Answer from the drawing. Dimensions are ordinates in mm from the lowest x, y and z of the part. Round coordinates to 2 decimals unless told otherwise and drop trailing zeros. Loops run counter-clockwise (first coordinate to the right, second up) from the corner with the lowest first, then second, coordinate; pieces in that order, holes last.
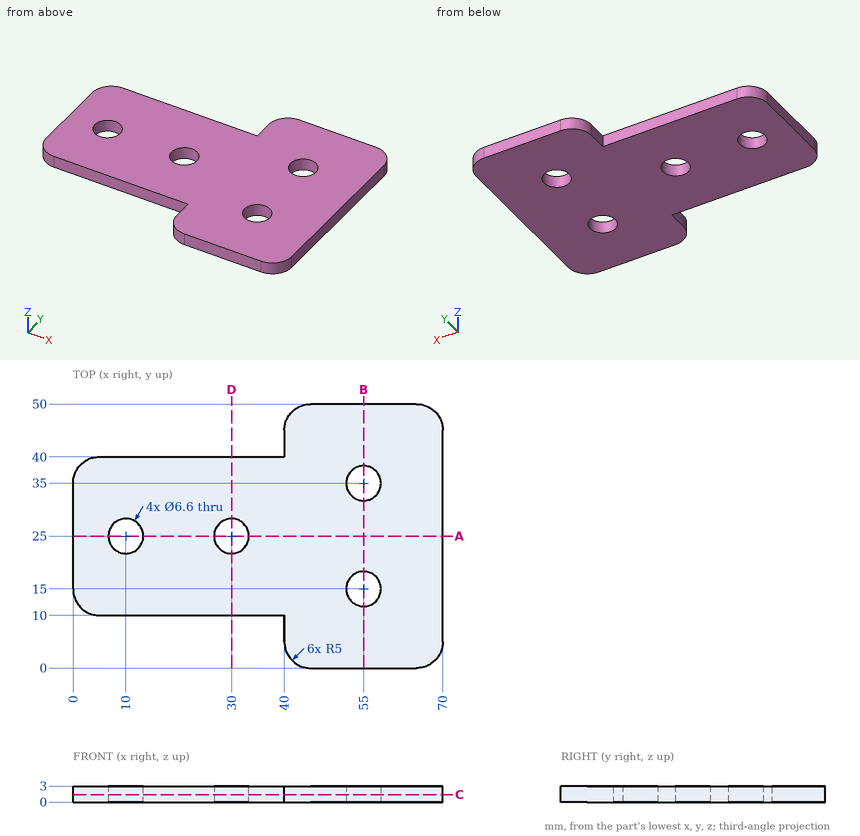
1. Find section D-D (x = 30). Write down the section's boundary in (y, z), then the cut area to 3 significant figures.
Answer key:
outline: (10, 0) - (21.7, 0) - (21.7, 3) - (10, 3) - close; (28.3, 0) - (40, 0) - (40, 3) - (28.3, 3) - close
area: 70.2 mm2
2. Find section A-A (y = 25). Write down the section's boundary in (x, z).
Answer key:
outline: (0, 0) - (6.7, 0) - (6.7, 3) - (0, 3) - close; (13.3, 0) - (26.7, 0) - (26.7, 3) - (13.3, 3) - close; (33.3, 0) - (70, 0) - (70, 3) - (33.3, 3) - close
3. Given pin 1 (10.5 mm diameter, centred on x = 55, y = 35, fed in from +Z); pin 2 (5.5 mm diameter, centred on x = 55, y = 15, fed in from -Z); pin 3 (1.5 mm diameter, centred on y = 7, z = 1, fed in from -X); pin 4 (1.5 mm diameter, centred on x = 17, z = 2.5, fed in from +Y), each flat-ended and moving along its own axis, determine where each tip first touches the part or whether it passes through.
Answer key:
pin 1: stops at z = 3
pin 2: passes through
pin 3: stops at x = 40
pin 4: stops at y = 40
4. Consider probe 1 along Y at (x, z) = (55, 1.1); probe 2 along Y at (x, z) = (10, 1.1); probe 3 along X at (y, z) = (28, 0.4). Determine where each line is inside the solid, lowest interval first.
Answer key:
probe 1: y = 0 to 11.7, 18.3 to 31.7, 38.3 to 50
probe 2: y = 10 to 21.7, 28.3 to 40
probe 3: x = 0 to 8.63, 11.37 to 28.63, 31.37 to 70
5. Find section B-B (x = 55). Write down the section's boundary in (y, z), then the cut area to 3 significant figures.
Answer key:
outline: (0, 0) - (11.7, 0) - (11.7, 3) - (0, 3) - close; (18.3, 0) - (31.7, 0) - (31.7, 3) - (18.3, 3) - close; (38.3, 0) - (50, 0) - (50, 3) - (38.3, 3) - close
area: 110 mm2
6. Find section C-C (z = 1.4). Write down the section's boundary in (x, y), then the cut area to 3 significant figures.
Answer key:
outline: (0, 15) arc R5 ccw to (5, 10) - (40, 10) - (40, 5) arc R5 ccw to (45, 0) - (65, 0) arc R5 ccw to (70, 5) - (70, 45) arc R5 ccw to (65, 50) - (45, 50) arc R5 ccw to (40, 45) - (40, 40) - (5, 40) arc R5 ccw to (0, 35) - close; hole circle Ø6.6 at (10, 25); hole circle Ø6.6 at (30, 25); hole circle Ø6.6 at (55, 15); hole circle Ø6.6 at (55, 35)
area: 2,530 mm2
